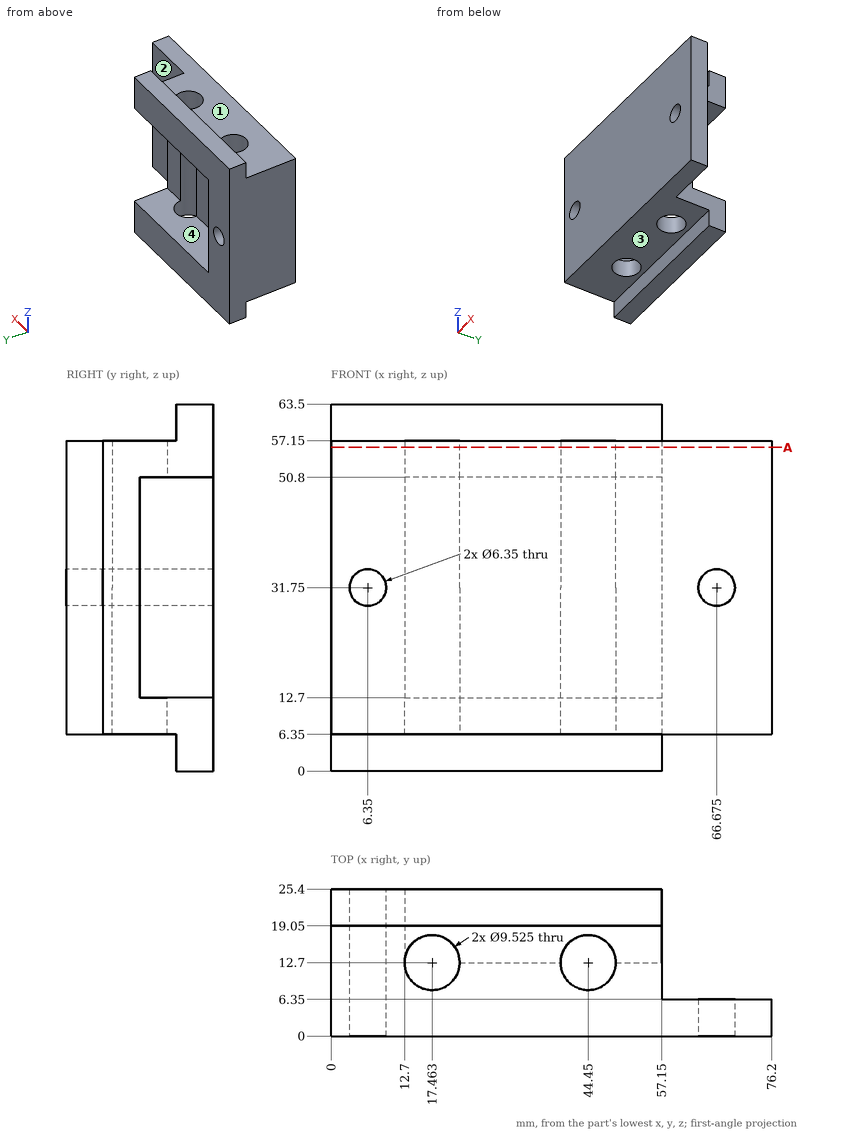
Part print with two shaded views. Sizes in mm from the minimum x, y, z corner. A direction names the side the tool comes from. Give positions to 0.01 mm unless a question says otherwise; leave off trailing zeros. Put each result on its own line as item: value.
Q1. Flat gauge pins, fed straight in: pin 1 (11 mm diameter, centred on x = 17.46, y = 12.7, fed in from -Z); pin 2 (8.5 mm diameter, centred on x = 44.45, y = 12.7, fed in from -Z); pin 3 (9.5 mm diameter, centred on x = 64, z = 40.5, fed in from +Y); pin 4 (15 mm diameter, centred on y = 20, z = 25, fed in from +X). Where does each tip first touch, or does it go through?
Filled in:
pin 1: stops at z = 6.35
pin 2: passes through
pin 3: stops at y = 6.35
pin 4: stops at x = 57.15
Q2. Tool access for the marked faces 1, 2, 3 and 4: list every direction of +Z, -Z, +X, -X, +Y, -Y with a clear straight run to the whole face (end or side of a thin tool).
Filled in:
face 1: +Z, +X, -X, -Y
face 2: +Z, -Z, +X, +Y
face 3: -Z, +X, -X, -Y
face 4: +X, +Y
Q3. Probe line 1 along Z through (x, y) = (14, 17.25); line 2 along Z through (x, y) = (20, 21); line 3 along X through (y, z) = (6.5, 54). List the from-to ranges inside material, lowest first.
Filled in:
line 1: z = 6.35 to 12.7, 50.8 to 57.15
line 2: z = 0 to 12.7, 50.8 to 63.5
line 3: x = 0 to 57.15
Q4. Slice it at A-A (z = 56). Give the number of separate pieces and of enclosed holes in the cut face, plus the area to 3 significant figures.
Filled in:
separate pieces: 1
enclosed holes: 2
area: 1,430 mm²
